Source: three-view drawing plus pictorial views. Frame: mm from the lowest corner of the part. A direction names the side the tool comes from. Give positions to 0.01 mm unless a question says otherwise; leave off trailing zeros. Order: outer loops, then holes, each group sorted by start corner. A loop starts at its lowest first (then second) coordinate and runs counter-clockwise, first axis right, second up. Notation, with made-up numbers: (-35.5, -24.5) - (-30.5, -24.5) arc R25 cw to (-30.5, -5.5) - close; hole circle Ø8 at (25.5, 87.25). An arc over 180 degrees is marked (long way). Use one line per item in the form item = value.
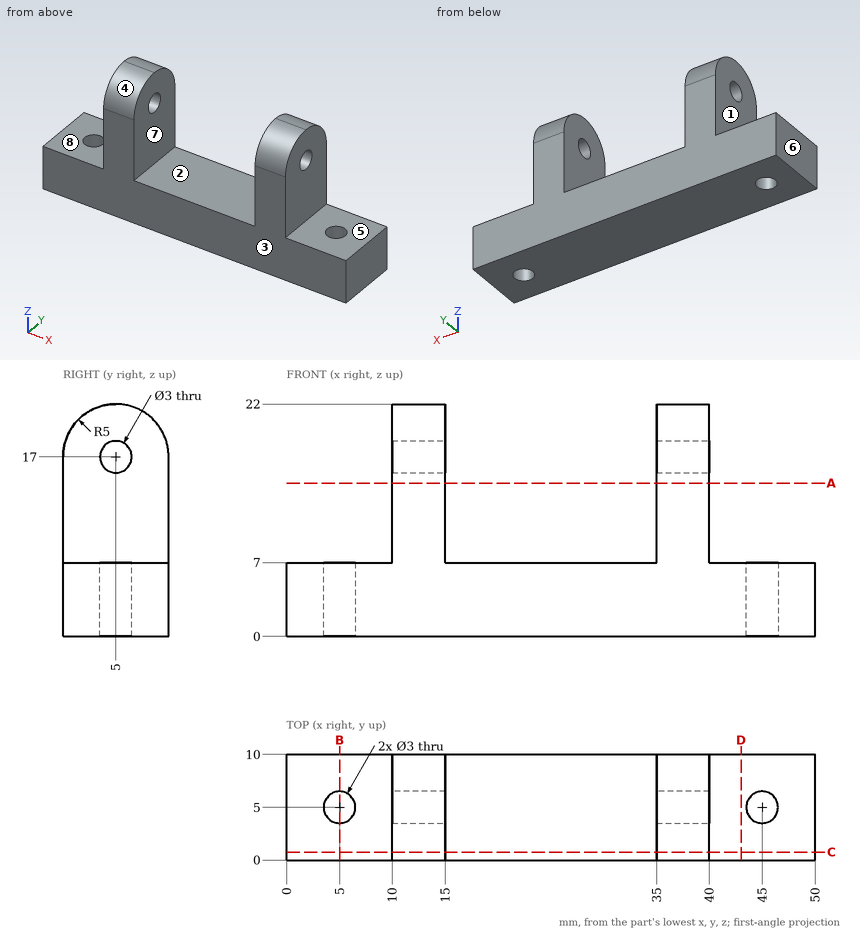
(1) Cut plane B-B on x = 5. Output: boundary loops of the cut face in (y, z).
Computed values:
outline = (0, 0) - (3.5, 0) - (3.5, 7) - (0, 7) - close; (6.5, 0) - (10, 0) - (10, 7) - (6.5, 7) - close
(2) Cut plane C-C on y = 0.75. Output: boundary loops of the cut face in (x, z), plus the area to 3 significant figures.
Computed values:
outline = (0, 0) - (50, 0) - (50, 7) - (40, 7) - (40, 19.63) - (35, 19.63) - (35, 7) - (15, 7) - (15, 19.63) - (10, 19.63) - (10, 7) - (0, 7) - close
area = 476 mm²
(3) Cut plane A-A on z = 14.5. Output: boundary loops of the cut face in (x, y).
Computed values:
outline = (10, 0) - (15, 0) - (15, 10) - (10, 10) - close; (35, 0) - (40, 0) - (40, 10) - (35, 10) - close
(4) Cut plane D-D on x = 43. Output: boundary loops of the cut face in (y, z), plus the area to 3 significant figures.
Computed values:
outline = (0, 0) - (10, 0) - (10, 7) - (0, 7) - close
area = 70.0 mm²
(5) Pull-direction query (X, two-part tool) for the marked faces 1, 2 and 3; classes: released by +X, released by -X, zero draft, split by the parting line, or undercut.
Computed values:
face_1 = released by -X
face_2 = undercut
face_3 = zero draft
(6) Contact query for flat-ended pins moving along their axis: pin 1 Ø3 at (y, z) = (6.5, 14) entering from +X; pin 2 Ø4 at (y, z) = (6, 19.5) entering from -X; pin 3 Ø3 at (x, y) = (47.5, 4.5) entering from +Z. Output: stop coordinate, or through.
Computed values:
pin_1 = 40
pin_2 = 10
pin_3 = 7
(7) Reachability of the marked faces 4, 5, 6, 7 and 8 from +Z, -Z, +X, -X, +Y, -Y: full face, straight path, thin tool, end or side. Return the list, or none.
Computed values:
face_4 = +Z, +X, -X, -Y
face_5 = +Z, +X, +Y, -Y
face_6 = +Z, -Z, -X, +Y, -Y
face_7 = +Z, +Y, -Y
face_8 = +Z, -X, +Y, -Y
(8) Ray query, line 1 along X through (y, z) = (2.5, 19.75); line 2 along Y through (x, z) = (45, 5.5); line 3 along Z through (x, y) = (46.5, 2.5). Return the intervals inside material, ascending.
Computed values:
line_1 = 10 to 15, 35 to 40
line_2 = 0 to 3.5, 6.5 to 10
line_3 = 0 to 7
